Read the model definition and answer for the solid it produces. Units are mm, in the model's axes. A direction names the side the tool comes from. Coordinates: 2 decimals unless noted, no trailing zeros. Order: outer loops, then holes, each group sorted by start corner. A loop starts at its lowest first (then second) coordinate and runs counter-clockwise, first axis right, second up.
from build123d import *

# Parameters (mm, degrees)
SKETCH1_R           = 90.17
BOSS_EXTRUDE1_DEPTH = 0.762
SKETCH2_R           = 69.85
BOSS_EXTRUDE2_DEPTH = 9.144
SKETCH3_R           = 41.402
BOSS_EXTRUDE3_DEPTH = 33.02
SKETCH4_R           = 19.1262
BOSS_EXTRUDE4_DEPTH = 7.62
SKETCH5_R           = 4.0005
BOSS_EXTRUDE5_DEPTH = 35.7632
CUT_EXTRUDE1_DEPTH  = 24.4602
SKETCH7_R           = 2.7178
CUT_EXTRUDE2_DEPTH  = 6.35
SKETCH8_R           = 2.1209
CUT_EXTRUDE3_DEPTH  = 6.35
SKETCH9_R           = 40.64
BOSS_EXTRUDE6_DEPTH = 50.8


with BuildPart() as part:
    # Sketch1 → Boss-Extrude1 (new, symmetric)
    with BuildSketch(Plane(origin=(0, 0, 0), x_dir=(1, 0, 0), z_dir=(0, 1, 0))):
        with Locations(Location((0, 0, 0), (0, 0, 90))):
            Circle(SKETCH1_R)
    extrude(amount=BOSS_EXTRUDE1_DEPTH, both=True)

    # Sketch2 → Boss-Extrude2 (add)
    with BuildSketch(Plane(origin=(0, 0.762, 0), x_dir=(1, 0, 0), z_dir=(0, 1, 0))):
        with Locations(Location((0, 0, 0), (0, 0, 270))):
            Circle(SKETCH2_R)
    extrude(amount=BOSS_EXTRUDE2_DEPTH)

    # Sketch3 → Boss-Extrude3 (add)
    with BuildSketch(Plane(origin=(0, 9.906, 0), x_dir=(1, 0, 0), z_dir=(0, 1, 0))):
        with Locations(Location((0, 0, 0), (0, 0, 270))):
            Circle(SKETCH3_R)
    extrude(amount=BOSS_EXTRUDE3_DEPTH)

    # Sketch4 → Boss-Extrude4 (add)
    with BuildSketch(Plane(origin=(0, 42.926, 0), x_dir=(1, 0, 0), z_dir=(0, 1, 0))):
        with Locations(Location((0, 0, 0), (0, 0, 90))):
            Circle(SKETCH4_R)
    extrude(amount=BOSS_EXTRUDE4_DEPTH)

    # Sketch5 → Boss-Extrude5 (add)
    with BuildSketch(Plane(origin=(0, 50.546, 0), x_dir=(1, 0, 0), z_dir=(0, 1, 0))):
        with Locations(Location((0, 0, 0), (0, 0, 270))):
            Circle(SKETCH5_R)
    extrude(amount=BOSS_EXTRUDE5_DEPTH)

    # Sketch6 → Cut-Extrude1 (cut)
    with BuildSketch(Plane(origin=(0, 86.3092, 0), x_dir=(1, 0, 0), z_dir=(0, 1, 0))):
        with BuildLine():
            Line((-3.0734, -2.6797), (-3.0734, 2.6797))
            ThreePointArc((-3.0734, 2.6797), (-4.077570312, 0), (-3.0734, -2.6797))
        make_face()
    extrude(amount=-CUT_EXTRUDE1_DEPTH, mode=Mode.SUBTRACT)

    # Sketch7 → Cut-Extrude2 (cut)
    with BuildSketch(Plane(origin=(0, 0.762, 0), x_dir=(1, 0, 0), z_dir=(0, 1, 0))):
        with Locations(Location((0, 85.1408, 0), (0, 0, 270))):
            Circle(SKETCH7_R)
        with Locations(Location((73.734095699, -42.5704, 0), (0, 0, 270))):
            Circle(SKETCH7_R)
        with Locations(Location((-73.734095699, -42.5704, 0), (0, 0, 270))):
            Circle(SKETCH7_R)
    extrude(amount=-CUT_EXTRUDE2_DEPTH, mode=Mode.SUBTRACT)

    # Sketch8 → Cut-Extrude3 (cut)
    with BuildSketch(Plane(origin=(0, 0.762, 0), x_dir=(1, 0, 0), z_dir=(0, 1, 0))):
        with Locations(Location((-81.657901206, 20.433276927, 0), (0, 0, 270))):
            Circle(SKETCH8_R)
        with Locations(Location((81.657901206, 20.433276927, 0), (0, 0, 270))):
            Circle(SKETCH8_R)
    extrude(amount=-CUT_EXTRUDE3_DEPTH, mode=Mode.SUBTRACT)

    # Sketch9 → Boss-Extrude6 (add)
    with BuildSketch(Plane.XZ.offset(0.762)):
        with Locations(Location((0, 0, 0), (0, 0, 90))):
            Circle(SKETCH9_R)
    extrude(amount=BOSS_EXTRUDE6_DEPTH)


solid = part.part
Q1. The part is cut by section D-D, the plane z = 34. Determine the outline of the cut face in (x, y), then the cut area to 3 significant figures.
Q2. The part is cut by section C-C, the plane y = -40.5. Determine the outline of the cut face in (x, z), then the cut area to 3 significant figures.
Q3. Determine the mould class of faces 1 (the flat face through (-3.073, 74, 0)), 2 (the cylindrical face through (-5.745, 46.683, -18.243)), 3 (the cylindrical face through (0.119, 0.011, -87.856)) for opening direction X: +X half, -X half, draft (parallel to the pull), parting line (faces both ways), or undercut.
Q4. Each of these flat-tipped pins is pushed along its axis until it touches: P1, Ø12, axis at y = 0.5, z = -59, coming from the +X side; P2, Ø1.5, axis at x = -25, y = -13.5, coming from the +Z side; P3, Ø1.5, axis at y = 78, z = 1, coming from the -X side; P4, Ø3.5, axis at x = 81.66, z = -20.43, coming from the -Y side. Where does it stop, or does it pass through?
Q5. Which of the six approach directions +Z, -Z, +X, -X, +Y, -Y give full straight-line access (tool end or side, diameter ignored) to faces 4 (the flat face through (39, -0.762, -19)), 5 (the flat face through (-9, 42.926, 18)), 6 (the cylindrical face through (71.08, 0.01, 41.98))?
Q6. The part is cut by section B-B, the plane z = 0. Determine the outline of the cut face in (x, y), then the cut area to 3 significant figures.
Q7. The part is cut by section A-A, the plane x = 0. Determine the outline of the cut face in (y, z).
Q8. Straight lines are drawn through the part: L1, parallel to Y at x = 23, z = 31; L2, parallel to X at y = -11, z = -1; L3, parallel to Y at x = -69.5, z = 46.5. For each, find the intervals that lie inside material, in ascending order.
Computed values:
1. outline: (-83.51, -0.76) - (-22.26, -0.76) - (-22.26, -51.56) - (22.26, -51.56) - (22.26, -0.76) - (83.51, -0.76) - (83.51, 0.76) - (61.02, 0.76) - (61.02, 9.91) - (23.62, 9.91) - (23.62, 42.93) - (-23.62, 42.93) - (-23.62, 9.91) - (-61.02, 9.91) - (-61.02, 0.76) - (-83.51, 0.76) - close
1. area: 5,190 mm2
2. outline: circle Ø81.28 at (0, 0)
2. area: 5,190 mm2
3. face 1: -X half
3. face 2: parting line
3. face 3: undercut
4. P1: stops at x = 72.95
4. P2: stops at z = 32.61
4. P3: stops at x = -3.07
4. P4: passes through
5. face 4: -Y
5. face 5: +Y
5. face 6: +Y, -Y
6. outline: (-90.17, -0.76) - (-40.64, -0.76) - (-40.64, -51.56) - (40.64, -51.56) - (40.64, -0.76) - (90.17, -0.76) - (90.17, 0.76) - (69.85, 0.76) - (69.85, 9.91) - (41.4, 9.91) - (41.4, 42.93) - (19.13, 42.93) - (19.13, 50.55) - (4, 50.55) - (4, 86.31) - (-3.07, 86.31) - (-3.07, 61.85) - (-4, 61.85) - (-4, 50.55) - (-19.13, 50.55) - (-19.13, 42.93) - (-41.4, 42.93) - (-41.4, 9.91) - (-69.85, 9.91) - (-69.85, 0.76) - (-90.17, 0.76) - close
6. area: 8,970 mm2
7. outline: (-51.56, -40.64) - (-0.76, -40.64) - (-0.76, -82.42) - (0.76, -82.42) - (0.76, -69.85) - (9.91, -69.85) - (9.91, -41.4) - (42.93, -41.4) - (42.93, -19.13) - (50.55, -19.13) - (50.55, -4) - (86.31, -4) - (86.31, 4) - (50.55, 4) - (50.55, 19.13) - (42.93, 19.13) - (42.93, 41.4) - (9.91, 41.4) - (9.91, 69.85) - (0.76, 69.85) - (0.76, 90.17) - (-0.76, 90.17) - (-0.76, 40.64) - (-51.56, 40.64) - close; (-0.76, -90.17) - (0.76, -90.17) - (0.76, -87.86) - (-0.76, -87.86) - close
8. L1: y = -51.56 to 42.93
8. L2: x = -40.63 to 40.63
8. L3: y = -0.76 to 0.76
